Autodesk Inventor part; units mm, degrees
ref_plane "YZ Plane" through (0, 0, 0) normal (1, 0, 0) x (0, 1, 0)
ref_plane "XZ Plane" through (0, 0, 0) normal (0, 1, 0) x (-1, 0, 0)
ref_plane "XY Plane" through (0, 0, 0) normal (0, 0, 1) x (1, 0, 0)
sketch "Sketch1" plane through (0, 0, 0) normal (0, 0, 1) x (1, 0, 0)
  line L0 (18.5838, -6.189) -> (18.5838, 42.8381)
  line L1 (18.5838, 42.8381) -> (12.2763, 47.2547)
  line L2 (12.2763, 47.2547) -> (-22.1957, 18.3292)
  line L3 (-22.1957, 18.3292) -> (-6.5665, -18.491)
  line L4 (18.5838, -6.189) -> (-6.5665, -18.491)
  point P0 (0, 0)
  point P1 (0, 0)
  dimension "d0" = 125
  dimension "d1" = 116.065
  dimension "d2" = 50
  dimension "d3" = 23
  dimension "d4" = 18.5838
  dimension "d5" = 45.7502
  dimension "d6" = 13.7251
  dimension "d7" = 28.3081
  dimension "d8" = 13.2695
extrude "Extrusion1" add sketch "Sketch1" against normal blind 3
properties part number "Tafe WA LOGO backplate"
The model under review builds one solid part; all positions refer to its coordinate system, in mm. Give positions to 0.01 mm unless a question says otherwise; leave off trailing zeros. Order: outer loops, then holes, each group sorted by start corner. A loop starts at its lowest first (then second) coordinate and runs counter-clockwise, first axis right, second up. Notation, with made-up numbers: (57.5, 71) - (115.5, 71) arc R32 cw to (115.5, 107) - close; hole circle Ø4 at (50.25, 78.5). An arc over 180 degrees is marked (long way). Use CSV: the item, a comma, the result in double quotes. Start each with the question number.
Q1. We need section C-C, the plane y = 7. Write out the cut boundary in (x, z).
Q2. We need section B-B, the plane x = -16. Write out the cut boundary in (y, z).
Q3. To check wall thickness, follow line 1 along Y through (x, z) = (-3.5, -0.15); line 2 along Y through (x, z) = (-5, -2.65); line 3 along X through (y, z) = (39, -1). State the ranges of each line that lie inside material, in increasing order. Write a range as [from, to].
Q4. We need section A-A, the plane z = -2. Write out the cut boundary in (x, y).
Q5. Clearance check with a flat-ended pin moving along its axis: pin 1 Ø1.5 at (x, z) = (4, -1.5) entering from -Y. State where the tip first meets the part, or that it passes through.
Outcome:
1,outline,"(-17.39, -3) - (18.58, -3) - (18.58, 0) - (-17.39, 0) - close"
2,outline,"(3.73, -3) - (23.53, -3) - (23.53, 0) - (3.73, 0) - close"
3,line 1,"y = [-16.99, 34.02]"
3,line 2,"y = [-17.72, 32.76]"
3,line 3,"x = [2.44, 18.58]"
4,outline,"(-22.2, 18.33) - (-6.57, -18.49) - (18.58, -6.19) - (18.58, 42.84) - (12.28, 47.25) - close"
5,pin 1,"stops at y = -13.69"
